Can you work these out from the model? Positions are in its coordinate system, mm. Face numbers are marked on the shaded views. A direction names the side the tool comes from. Round coordinates to 2 decimals unless told otherwise and drop trailing zeros. Loops run counter-clockwise (first coordinate to the right, second up) from the corner with the lowest first, then second, coordinate; pieces in that order, holes last.
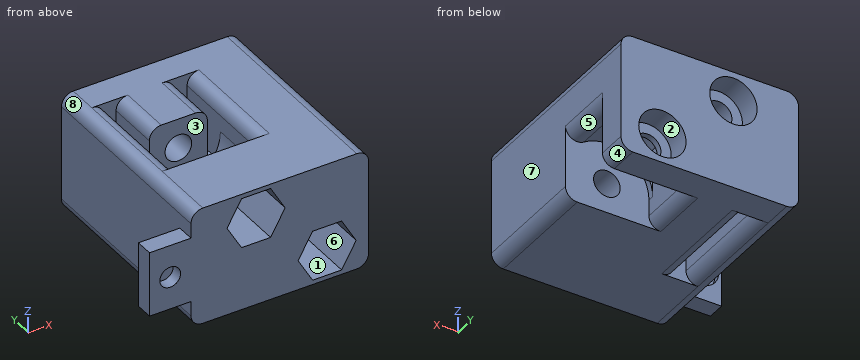
from build123d import *

# Parameters (mm, degrees)
SKETCH1_W                                           = 30
SKETCH1_H                                           = 20
BOSS_EXTRUDE1_DEPTH                                 = 11
SKETCH2_W                                           = 4
SKETCH2_H                                           = 20
BOSS_EXTRUDE2_DEPTH                                 = 19
SKETCH3_W                                           = 30
SKETCH3_H                                           = 20
BOSS_EXTRUDE3_DEPTH                                 = 5
BOSS_EXTRUDE4_START                                 = 9
BOSS_EXTRUDE4_DEPTH                                 = 9
BOSS_EXTRUDE5_DEPTH                                 = 9
BOSS_EXTRUDE6_DEPTH                                 = 1
FILLET1_R                                           = 2
SKETCH7_R                                           = 2.25
CUT_EXTRUDE1_DEPTH                                  = 40.37003937
CBORE_FOR_M4_HEX_SOCKET_HEAD_CAP_SCREW2_D           = 4.5
CBORE_FOR_M4_HEX_SOCKET_HEAD_CAP_SCREW2_CBORE_D     = 8
CBORE_FOR_M4_HEX_SOCKET_HEAD_CAP_SCREW2_CBORE_DEPTH = 4
CUT_EXTRUDE4_DEPTH                                  = 10
SKETCH23_W                                          = 11
SKETCH23_H                                          = 3
BOSS_EXTRUDE10_DEPTH                                = 7
SKETCH24_R                                          = 1.75
CUT_EXTRUDE7_DEPTH                                  = 7
SKETCH25_R                                          = 3
CUT_EXTRUDE8_DEPTH                                  = 1
FILLET2_R                                           = 2


with BuildPart() as part:
    # Sketch1 → Boss-Extrude1 (new body)
    with BuildSketch(Plane(origin=(0, 0, 0), x_dir=(1, 0, 0), z_dir=(0, 1, 0))):
        Rectangle(SKETCH1_W, SKETCH1_H)
    extrude(amount=BOSS_EXTRUDE1_DEPTH)

    # Sketch2 → Boss-Extrude2 (add)
    with BuildSketch(Plane(origin=(0, 11, 0), x_dir=(1, 0, 0), z_dir=(0, 1, 0))):
        with Locations((-13, 0)):
            Rectangle(SKETCH2_W, SKETCH2_H)
        with BuildLine():
            Line((0.898979486, 10), (-8.898979486, 10))
            Line((-8.898979486, 10), (-8.898979486, 0))
            ThreePointArc((-8.898979486, 0), (-4, 2), (0.898979486, 0))
            Line((0.898979486, 0), (0.898979486, 10))
        make_face()
        with BuildLine():
            Line((3.101020514, 0), (3.101020514, -10))
            Line((3.101020514, -10), (15, -10))
            Line((15, -10), (15, 5))
            ThreePointArc((15, 5), (10.711747002, -1.453404388), (3.101020514, 0))
        make_face()
    extrude(amount=BOSS_EXTRUDE2_DEPTH)

    # Sketch3 → Boss-Extrude3 (add)
    with BuildSketch(Plane(origin=(0, 30, 0), x_dir=(1, 0, 0), z_dir=(0, 1, 0))):
        Rectangle(SKETCH3_W, SKETCH3_H)
    extrude(amount=BOSS_EXTRUDE3_DEPTH)

    # Sketch4 → Boss-Extrude4 (add)
    with BuildSketch(Plane.XZ.offset(-30).offset(BOSS_EXTRUDE4_START)):
        with BuildLine():
            Line((-8.898979486, 0), (-8.898979486, 10))
            Line((-8.898979486, 10), (0.898979486, 10))
            Line((0.898979486, 10), (0.898979486, 0))
            ThreePointArc((0.898979486, 0), (-4, -2), (-8.898979486, 0))
        make_face()
    extrude(amount=-BOSS_EXTRUDE4_DEPTH)

    # Sketch5 → Boss-Extrude5 (add)
    with BuildSketch(Plane(origin=(0, 11, 0), x_dir=(1, 0, 0), z_dir=(0, 1, 0))):
        with BuildLine():
            Line((15, 10), (15, 5))
            ThreePointArc((15, 5), (10.711747002, -1.453404388), (3.101020514, 0))
            Line((3.101020514, 0), (3.101020514, -5.240408206))
            ThreePointArc((3.101020514, -5.240408206), (2.528143689, -2.398275958), (0.898979486, 0))
            Line((0.898979486, 0), (0.898979486, 10))
            Line((0.898979486, 10), (15, 10))
        make_face()
    extrude(amount=BOSS_EXTRUDE5_DEPTH)

    # Sketch6 → Boss-Extrude6 (add)
    with BuildSketch(Plane(origin=(0, 20, 0), x_dir=(1, 0, 0), z_dir=(0, 1, 0))):
        with BuildLine():
            Line((3.101020514, 0), (3.101020514, -5.240408206))
            ThreePointArc((3.101020514, -5.240408206), (2.528143689, -2.398275958), (0.898979486, 0))
            Line((0.898979486, 0), (0.898979486, 5.240408206))
            ThreePointArc((0.898979486, 5.240408206), (1.471856311, 2.398275958), (3.101020514, 0))
        make_face()
    extrude(amount=BOSS_EXTRUDE6_DEPTH)

    # Fillet1
    fillet1_edges = [part.edges().sort_by_distance(p)[0] for p in [
        (-11, 20.5, 10),
        (-11, 20.5, -10),
        (0.898979486, 25, -10),
        (-8.898979486, 20.5, -10),
        (15, 25, -5),
        (3.101020514, 20.5, 10),
        (0.898979486, 25.5, 10),
        (-8.898979486, 25.5, 10),
    ]]
    fillet(fillet1_edges, radius=FILLET1_R)

    # Sketch7 → Cut-Extrude1 (cut, through all)
    with BuildSketch(Plane(origin=(0, 35, 0), x_dir=(1, 0, 0), z_dir=(0, 1, 0))):
        with Locations(Location((-4, -5, 0), (0, 0, 270))):
            Circle(SKETCH7_R)
        with Locations(Location((8, 5, 0), (0, 0, 270))):
            Circle(SKETCH7_R)
    extrude(amount=-CUT_EXTRUDE1_DEPTH, mode=Mode.SUBTRACT)

    # CBORE for M4 Hex Socket Head Cap Screw2 (through all)
    with Locations(Plane(origin=(0, 35, 0), x_dir=(1, 0, 0), z_dir=(0, 1, 0))):
        with Locations((-4, -5), (8, 5)):
            CounterBoreHole(CBORE_FOR_M4_HEX_SOCKET_HEAD_CAP_SCREW2_D / 2, CBORE_FOR_M4_HEX_SOCKET_HEAD_CAP_SCREW2_CBORE_D / 2, CBORE_FOR_M4_HEX_SOCKET_HEAD_CAP_SCREW2_CBORE_DEPTH)

    # Sketch12 → Cut-Extrude4 (cut)
    with BuildSketch(Plane.XZ):
        Polygon((0.907477288, 5), (-1.546261356, 9.25), (-6.453738644, 9.25), (-8.907477288, 5), (-6.453738644, 0.75), (-1.546261356, 0.75), align=None)
        Polygon((3.092522712, -5), (5.546261356, -9.25), (10.453738644, -9.25), (12.907477288, -5), (10.453738644, -0.75), (5.546261356, -0.75), align=None)
    extrude(amount=-CUT_EXTRUDE4_DEPTH, mode=Mode.SUBTRACT)

    # Sketch23 → Boss-Extrude10 (add)
    with BuildSketch(Plane.ZY.offset(15)):
        with Locations((0, 1.5)):
            Rectangle(SKETCH23_W, SKETCH23_H)
    extrude(amount=BOSS_EXTRUDE10_DEPTH)

    # Sketch24 → Cut-Extrude7 (cut)
    with BuildSketch(Plane(origin=(0, 3, 0), x_dir=(1, 0, 0), z_dir=(0, 1, 0))):
        with Locations(Location((-18.5, 0, 0), (0, 0, 270))):
            Circle(SKETCH24_R)
    extrude(amount=-CUT_EXTRUDE7_DEPTH, mode=Mode.SUBTRACT)

    # Sketch25 → Cut-Extrude8 (cut)
    with BuildSketch(Plane(origin=(0, 3, 0), x_dir=(1, 0, 0), z_dir=(0, 1, 0))):
        with Locations(Location((-18.5, 0, 0), (0, 0, 270))):
            Circle(SKETCH25_R)
    extrude(amount=-CUT_EXTRUDE8_DEPTH, mode=Mode.SUBTRACT)

    # Fillet2
    fillet2_edges = [part.edges().sort_by_distance(p)[0] for p in [
        (15, 32.5, -10),
        (15, 17.5, 10),
        (-15, 17.5, 10),
        (-15, 17.5, -10),
        (15, 10, -10),
    ]]
    fillet(fillet2_edges, radius=FILLET2_R - 0.0001)  # a hair under: the kernel refuses the full size


solid = part.part
(1) Will these pins go through, and if not, where does the flat tip stop? P1, Ø1, axis at x = -15, y = 5, coming from the +Z side; P2, Ø5, axis at x = -4, z = 5, coming from the -Y side; P3, Ø5, axis at y = 16.5, z = -5, coming from the -X side; P4, Ø3, axis at x = -18.5, z = 0, coming from the -Y side.
Worked answers:
P1: stops at z = 9.32
P2: stops at y = 10
P3: stops at x = -15
P4: passes through
(2) If we section it at C-C, the plane x = -18.5: List the corners of the cut face in (y, z) for me, then the cut area to 3 significant figures.
Worked answers:
outline: (0, -5.5) - (3, -5.5) - (3, -3) - (2, -3) - (2, -1.75) - (0, -1.75) - close; (0, 1.75) - (2, 1.75) - (2, 3) - (3, 3) - (3, 5.5) - (0, 5.5) - close
area: 20.0 mm2
(3) If we mould it in two halves opening along Z, with no side actions, what happens to the marked faces 6, 7 and 8? For each: released by +Z, released by -Z, zero draft, split by the parting line, or undercut.
Worked answers:
face 6: undercut
face 7: zero draft
face 8: released by +Z
(4) If I drill on line 1 (X direction, y = 17.5, z = -5); line 2 (Z direction, x = -4, y = 31.9); line 3 (X direction, y = 0.65, z = 0), over which ranges is the centre line in solid material (lowest first)?
Worked answers:
line 1: x = -15 to -11, -8.9 to 5.75, 10.25 to 15
line 2: z = -10 to 1, 9 to 10
line 3: x = -22 to -20.25, -16.75 to 15
(5) For the marked faces 1, 2, 3, 4 and 5, which set-ups out of +Z, -Z, +X, -X, +Y, -Y let a thin tool reach every point of the face, with its end or its side?
Worked answers:
face 1: -Y
face 2: +Y
face 3: +Z
face 4: -Z, +X, +Y, -Y
face 5: -Z
(6) If we section it at B-B, the plane y = 8: List the corners of the cut face in (x, z) for me, then the cut area to 3 significant figures.
Worked answers:
outline: (-15, -8) arc R2 ccw to (-13, -10) - (13, -10) arc R2 ccw to (15, -8) - (15, 8) arc R2 ccw to (13, 10) - (-13, 10) arc R2 ccw to (-15, 8) - close; hole (-8.91, 5) - (-6.45, 0.75) - (-1.55, 0.75) - (0.91, 5) - (-1.55, 9.25) - (-6.45, 9.25) - close; hole (3.09, -5) - (5.55, -9.25) - (10.45, -9.25) - (12.91, -5) - (10.45, -0.75) - (5.55, -0.75) - close
area: 471 mm2
(7) If we section it at A-A, the plane x = -4: List the corners of the cut face in (y, z) for me, then the cut area to 4 significant figures.
Worked answers:
outline: (0, -10) - (35, -10) - (35, 1) - (31, 1) - (31, 2.75) - (21, 2.75) - (21, -2) - (11, -2) - (11, 2.75) - (10, 2.75) - (10, 0.75) - (0, 0.75) - close; (0, 9.25) - (10, 9.25) - (10, 7.25) - (11, 7.25) - (11, 10) - (0, 10) - close; (21, 7.25) - (31, 7.25) - (31, 9) - (35, 9) - (35, 10) - (21, 10) - close
area: 413.5 mm2
